Autodesk Inventor part; units mm, degrees
ref_plane "YZ Plane" through (0, 0, 0) normal (1, 0, 0) x (0, 1, 0)
ref_plane "XZ Plane" through (0, 0, 0) normal (0, 1, 0) x (-1, 0, 0)
ref_plane "XY Plane" through (0, 0, 0) normal (0, 0, 1) x (1, 0, 0)
sketch "Sketch1" plane through (0, 0, 0) normal (0, 0, 1) x (1, 0, 0)
  line L0 (0, 0) -> (-100, 0)
  line L1 (-100, 0) -> (-100, 100)
  line L2 (-100, 100) -> (0, 100)
  line L3 (0, 100) -> (0, 0)
  dimension "d0" = 100
  dimension "d1" = 100
extrude "Extrusion1" add sketch "Sketch1" along normal blind 5
sketch "Sketch11" plane through (-80, 15, 0) normal (0, 0, -1) x (-1, 0, 0)
  circle A0 centre (0, 0) radius 3.3
  circle A1 centre (-30, 0) radius 5
  circle A2 centre (-30, 0) radius 3
  circle A3 centre (-60, 0) radius 5
  circle A4 centre (-60, 0) radius 3.3
  point P0 (-80, -15)
  dimension "d101" = 6.6
  dimension "d102" = 6
  dimension "d103" = 6.6
extrude "Extrusion11" cut sketch "Sketch11" along normal through all both and the other way through all contours A0 | A4
sketch "Sketch7" plane through (0, 0, 0) normal (0, 0, -1) x (-1, 0, 0)
  line L0 (100, 25) -> (0, 25)
  line L1 (100, 56.2495) -> (100, 25)
  line L2 (100, 100) -> (0, 100)
  line L3 (0, 0) -> (100, 0)
  circle A0 centre (86.5, 88) radius 4
  circle A1 centre (86.5, 88) radius 1.65
  line L4 (50, 100) -> (50, 0)
  line L5 (100, 0) -> (0, 0)
  line L6 (0, 100) -> (0, 100)
  line L7 (0, 100) -> (0, 98.5)
  circle A2 centre (95, 95) radius 2.5
  line L8 (100, 0) -> (100, 100)
  line L9 (0, 0) -> (100, 0)
  line L10 (100, 0) -> (100, 100)
  line L11 (100, 100) -> (0, 100)
  line L12 (0, 100) -> (0, 0)
  circle A3 centre (13.5, 88) radius 4
  circle A4 centre (13.5, 88) radius 1.65
  circle A5 centre (5, 95) radius 2.5
  point P0 (95.4835, 97.4528)
  point P1 (95.4244, 97.4637)
  point P2 (0, 100)
  point P3 (0, 100)
  point P4 (4.5165, 97.4528)
  point P5 (4.5756, 97.4637)
  point P6 (0, 100)
  dimension "d72" = 25
  dimension "d77" = 8
  dimension "d78" = 3.3
  dimension "d88" = 5
  dimension "d111" = 5
  dimension "d112" = 8.5
  dimension "d121" = 7
  dimension "d122" = 5
extrude "Extrusion13" cut sketch "Sketch7" against normal blind 10 contours A0 | A1 | A2 | A3 | A4 | A5
sketch "Sketch13" plane through (0, 0, 5) normal (0, 0, 1) x (1, 0, 0)
  line L0 (-10, 25) -> (-90, 25) construction
  line L1 (-90, 25) -> (-90, 85) construction
  line L2 (-90, 85) -> (-10, 85) construction
  line L3 (-10, 85) -> (-10, 25) construction
  line L4 (0, 0) -> (0, 100)
  line L5 (-100, 100) -> (-100, 0)
  line L6 (-100, 0) -> (0, 0)
  dimension "d123" = 10
  dimension "d124" = 80
  dimension "d125" = 60
  dimension "d126" = 100
  dimension "d127" = 25
equation "\"d103\" = d101"
equation "\"d88\" = d86"
equation "\"d123\" = -0.5 * d124 + 0.5 * d126"
properties part number "PlaqueGuideBlocLame" material "Aluminum 6061"
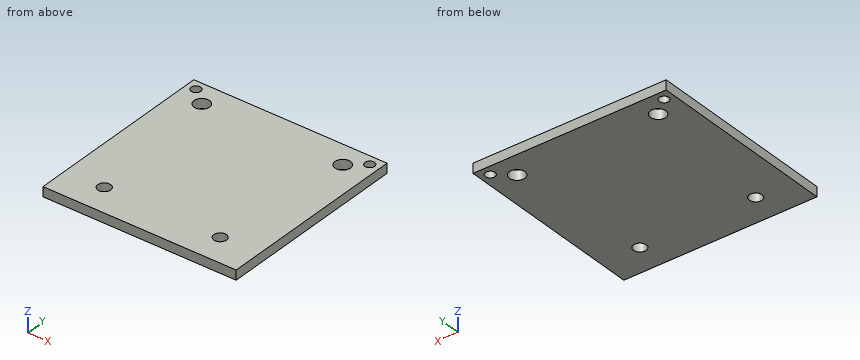
Work out the finished part from the listing and answer in its coordinate system (mm). Give positions to 0.01 mm unless a question says otherwise; leave off trailing zeros. Order: outer loops, then holes, each group sorted by start corner. A loop starts at its lowest first (then second) coordinate and runs counter-clockwise, first axis right, second up. Notation, with made-up numbers: (-31, -35) - (-9, -35) arc R26 cw to (-9, -1) - close; hole circle Ø5 at (-9, 2). An arc over 180 degrees is marked (long way). One line per item, written item: value. Start each with the question number.
1. Consider line 1 (Y direction, x = -5, z = 1.5); line 2 (Y direction, x = -20, z = 1.85). Determine where each line is inside the solid, lowest interval first.
2. Section C-C, the plane z = 3.55 is taken. Write down the section's boundary in (x, y).
3. Section D-D, the plane y = 15 is taken. Write down the section's boundary in (x, z).
4. Section B-B, the plane y = 88 is taken. Write down the section's boundary in (x, z), then the cut area to 3 significant figures.
5. Section A-A, the plane x = -95 is taken. Write down the section's boundary in (y, z).
6. This flat-tipped pin is pushed along its axis until it touches: pin 1 Ø1.5 at (x, z) = (-61, 0.5) entering from -Y. Where does it stop, or does it pass through?
Filled sheet:
1. line 1: 0 to 92.5, 97.5 to 100
1. line 2: 0 to 11.7, 18.3 to 100
2. outline: (-100, 0) - (0, 0) - (0, 100) - (-100, 100) - close; hole circle Ø5 at (-95, 95); hole circle Ø8 at (-86.5, 88); hole circle Ø6.6 at (-80, 15); hole circle Ø6.6 at (-20, 15); hole circle Ø8 at (-13.5, 88); hole circle Ø5 at (-5, 95)
3. outline: (-100, 0) - (-83.3, 0) - (-83.3, 5) - (-100, 5) - close; (-76.7, 0) - (-23.3, 0) - (-23.3, 5) - (-76.7, 5) - close; (-16.7, 0) - (0, 0) - (0, 5) - (-16.7, 5) - close
4. outline: (-100, 0) - (-90.5, 0) - (-90.5, 5) - (-100, 5) - close; (-82.5, 0) - (-17.5, 0) - (-17.5, 5) - (-82.5, 5) - close; (-9.5, 0) - (0, 0) - (0, 5) - (-9.5, 5) - close
4. area: 420 mm²
5. outline: (0, 0) - (92.5, 0) - (92.5, 5) - (0, 5) - close; (97.5, 0) - (100, 0) - (100, 5) - (97.5, 5) - close
6. pin 1: y = 0
